The listing builds one solid part. Answer for the finished solid, in the listing's coordinates (mm). A direction names the side the tool comes from. Round coordinates to 2 decimals unless told otherwise and drop trailing zeros. Loops run counter-clockwise (first coordinate to the right, second up) from the corner with the lowest first, then second, coordinate; pieces in that order, holes last. Notation, with made-up numbers: (-9, 8.25) -> (16, 8.25) arc R19 ccw to (16, 40.25) -> close; hole circle Ø11 at (-18.5, 27). An arc over 180 degrees is marked (long way). Write each question's results on one line, items separated by ' | '. Start each with the question number.
(1) Straight lines are drawn through the part: probe 1 along X at (y, z) = (2.9, 5.75); probe 2 along Z at (x, y) = (-1.5, 1.8); probe 3 along Z at (x, y) = (-1.75, 0.7). For each, find the intervals that lie inside material, in ascending order.
(2) The part is cut by section A-A (z = 4). Determine the outline of the cut face in (x, y).
(3) The part is cut by section D-D (z = -1.25). Determine the outline of the cut face in (x, y), plus the area to 3 significant figures.
(4) Determine the mould class of faces 5 (the face through (5.57, 2.03, -8.4)), 6 (the face through (-5.86, 2.03, 0.82)), 7 (the face through (-6, 2, 7)) for opening direction Z: released by +Z, released by -Z, zero draft, split by the parting line, or undercut.
(5) For faces 1 (the face through (0, 2, -2)), 2 (the face through (1.6, 2, -8.4)), 3 (the face through (-5.83, 2.03, -4.1)), 4 (the face through (5.86, 2.03, 0.82)), determine the directions among +Z, -Z, +X, -X, +Y, -Y from which every point of the face is accessible in a straight line to the end or side of a thin tool.
(6) The part is cut by section B-B (x = -0.5). Determine the outline of the cut face in (y, z).
(7) Flat-ended cylindrical pins translate along their axes: pin 1 (4 mm diameter, centred on x = -3, z = -2, fed in from -Y); pin 2 (1.2 mm diameter, centred on y = 2, z = 4.5, fed in from +X); pin 3 (1.9 mm diameter, centred on y = 2, z = 3, fed in from -X); pin 4 (1.1 mm diameter, centred on x = 0.5, y = 1.5, fed in from -Z). Find the tip coordinate at first contact, or state that the pin passes through.
(8) The part is cut by section C-C (z = -6.75). Determine the outline of the cut face in (x, y) (3 decimals), plus the area to 3 significant figures.
```python
from build123d import *

# Parameters (mm, degrees)
BOSS_EXTRUDE2_DEPTH = 4
FILLET1_R           = 10
FILLET2_R           = 2.15
FILLET3_R           = 1.5


with BuildPart() as part:
    # Sketch1 → Boss-Extrude2 (new body)
    with BuildSketch(Plane(origin=(0, 0, 0), x_dir=(1, 0, 0), z_dir=(0, 1, 0))):
        with BuildLine():
            Line((6, -1.25), (6, 1.25))
            ThreePointArc((6, 1.25), (5.25, 2), (6, 2.75))
            Line((6, 2.75), (6, 8.85))
            Line((6, 8.85), (1.85, 8.85))
            ThreePointArc((1.85, 8.85), (1.172875656, 7.35), (1.85, 5.85))
            Line((1.85, 5.85), (1.85, 2))
            Line((1.85, 2), (-1.85, 2))
            Line((-1.85, 2), (-1.85, 5.85))
            ThreePointArc((-1.85, 5.85), (-1.172875656, 7.35), (-1.85, 8.85))
            Line((-1.85, 8.85), (-6, 8.85))
            Line((-6, 8.85), (-6, 2.75))
            ThreePointArc((-6, 2.75), (-5.25, 2), (-6, 1.25))
            Line((-6, 1.25), (-6, -1.25))
            ThreePointArc((-6, -1.25), (-5.25, -2), (-6, -2.75))
            Line((-6, -2.75), (-6, -8.85))
            Line((-6, -8.85), (-1.85, -8.85))
            ThreePointArc((-1.85, -8.85), (-1.172875656, -7.35), (-1.85, -5.85))
            Line((-1.85, -5.85), (-1.85, -2))
            Line((-1.85, -2), (1.85, -2))
            Line((1.85, -2), (1.85, -5.85))
            ThreePointArc((1.85, -5.85), (1.172875656, -7.35), (1.85, -8.85))
            Line((1.85, -8.85), (6, -8.85))
            Line((6, -8.85), (6, -2.75))
            ThreePointArc((6, -2.75), (5.25, -2), (6, -1.25))
        make_face()
    extrude(amount=BOSS_EXTRUDE2_DEPTH)

    # Fillet1
    fillet1_edges = [part.edges().sort_by_distance(p)[0] for p in [
        (-6, 2, 2.75),
        (-6, 2, -2.75),
        (6, 2, -2.75),
        (6, 2, 2.75),
    ]]
    fillet(fillet1_edges, radius=FILLET1_R)

    # Fillet2
    fillet2_edges = [part.edges().sort_by_distance(p)[0] for p in [
        (-6, 2, 1.25),
        (-6, 2, -1.25),
        (6, 2, -1.25),
        (6, 2, 1.25),
    ]]
    fillet(fillet2_edges, radius=FILLET2_R)

    # Fillet3
    fillet3_edges = [part.edges().sort_by_distance(p)[0] for p in [
        (-1.85, 2, 8.85),
        (-6, 2, 8.85),
        (-6, 2, -8.85),
        (-1.85, 2, -8.85),
        (1.85, 2, -8.85),
        (6, 2, -8.85),
        (6, 2, 8.85),
        (1.85, 2, 8.85),
    ]]
    fillet(fillet3_edges, radius=FILLET3_R)


solid = part.part
```
Checked values:
1) probe 1: x = -6 to -1.85, 1.85 to 6 | probe 2: z = -8.29 to -6.25, -2 to 2, 6.25 to 8.29 | probe 3: z = -8.53 to -5.94, -2 to 2, 5.94 to 8.53
2) outline: (-5.81, 0) -> (-1.85, 0) -> (-1.85, 4) -> (-5.81, 4) -> close; (1.85, 0) -> (5.81, 0) -> (5.81, 4) -> (1.85, 4) -> close
3) outline: (-5.64, 0) -> (5.64, 0) -> (5.64, 4) -> (-5.64, 4) -> close | area: 45.1 mm2
4) face 5: released by -Z | face 6: undercut | face 7: zero draft
5) face 1: +Y, -Y | face 2: -Z, +Y, -Y | face 3: -X, +Y, -Y | face 4: +X, +Y, -Y
6) outline: (0, -2) -> (4, -2) -> (4, 2) -> (0, 2) -> close
7) pin 1: stops at y = 0 | pin 2: stops at x = 5.96 | pin 3: stops at x = -5.8 | pin 4: stops at z = -2
8) outline: (-6, 0) -> (-1.265, 0) -> (-1.265, 4) -> (-6, 4) -> close; (1.265, 0) -> (6, 0) -> (6, 4) -> (1.265, 4) -> close | area: 37.9 mm2
